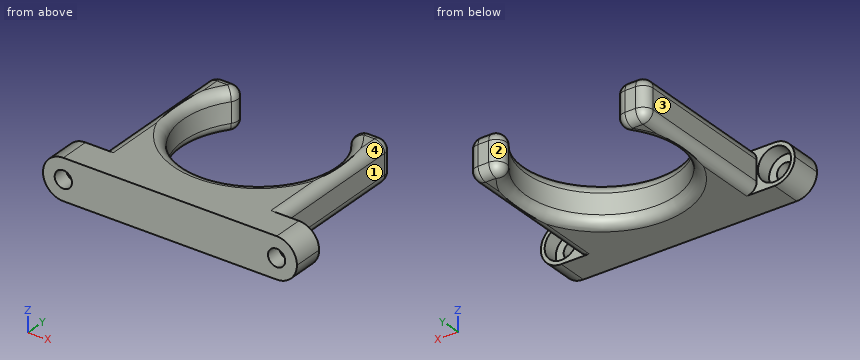
```python
from build123d import *

# Parameters (mm, degrees)
F1_DEPTH             = 8
F4_D                 = 3.4
F4_CBORE_D           = 6.5
F4_CBORE_DEPTH       = 3
F4_ON_F3_D           = 3.4
F4_ON_F3_CBORE_D     = 6.5
F4_ON_F3_CBORE_DEPTH = 3
F5_T1_DEPTH          = 2.0779215299
F5_T3_DEPTH          = 28
F5_T5_DEPTH          = 2.0779215299
F5_T8_ANGLE          = 253.4876833877
F5_T10_ANGLE         = 253.4876833877
F5_T12_ANGLE         = 126.7438416939
F5_T14_ANGLE         = 126.7438416939
F5_T16_ANGLE         = 90
F5_T18_ANGLE         = 90
F5_T20_ANGLE         = 126.7438416939
F5_T22_ANGLE         = 126.7438416939
F5_T24_ANGLE         = 90
F5_T26_ANGLE         = 90
F6_R                 = 3.99999


# Not quite as in the source:
# - a fillet or chamfer that OpenCascade refuses, or shapes differently, is made with other operations: its cross-section is extruded or revolved along the edge and cut away or added
# - a fillet or chamfer is up to 0.001 mm smaller than in the source, because OpenCascade refuses the exact size


with BuildPart() as f1:
    # F0 (on Top) → F1 (new body)
    with BuildSketch(Plane.XY):
        Polygon((-25, 6), (-25, 0), (25, 0), (25, 6), (17.5, 6), (-17.5, 6), align=None)
        with BuildLine():
            Line((-17.5, 34), (-17.5, 6))
            Line((-17.5, 6), (17.5, 6))
            Line((17.5, 6), (17.5, 34))
            ThreePointArc((17.5, 34), (16.9142135624, 35.4142135624), (15.5, 36))
            Line((15.5, 36), (13.4220784701, 36))
            ThreePointArc((13.4220784701, 36), (11.634209081, 34.896394471), (11.8194422349, 32.8035230476))
            ThreePointArc((11.8194422349, 32.8035230476), (0, 9.229505524), (-11.8194422349, 32.8035230476))
            ThreePointArc((-11.8194422349, 32.8035230476), (-11.634209081, 34.896394471), (-13.4220784701, 36))
            Line((-13.4220784701, 36), (-15.5, 36))
            ThreePointArc((-15.5, 36), (-16.9142135624, 35.4142135624), (-17.5, 34))
        make_face()
    extrude(amount=F1_DEPTH)

    # F4 (through all)
    with Locations(Plane(origin=(0, 6, 0), x_dir=(-1, 0, 0), z_dir=(0, 1, 0))):
        with Locations((-21, 4)):
            CounterBoreHole(F4_D / 2, F4_CBORE_D / 2, F4_CBORE_DEPTH)

    # F4 on F3 (through all)
    with Locations(Plane(origin=(0, 6, 0), x_dir=(-1, 0, 0), z_dir=(0, 1, 0))):
        with Locations((21, 4)):
            CounterBoreHole(F4_ON_F3_D / 2, F4_ON_F3_CBORE_D / 2, F4_ON_F3_CBORE_DEPTH)

    # F5: fillet of radius 2 on 2 edges, made by hand

    # F5_s2 → F5_t1 (cut)
    with BuildSketch(Plane.YZ.offset(-15.5)):
        with BuildLine():
            ThreePointArc((34, 8), (35.4142135624, 7.4142135624), (36, 6))
            Line((36, 6), (36, 8))
            Line((36, 8), (34, 8))
        make_face()
        with BuildLine():
            ThreePointArc((34, 0), (35.4142135624, 0.5857864376), (36, 2))
            Line((36, 2), (36, 0))
            Line((36, 0), (34, 0))
        make_face()
    extrude(amount=F5_T1_DEPTH, mode=Mode.SUBTRACT)

    # F5_s4 → F5_t3 (cut)
    with BuildSketch(Plane.XZ.offset(-34)):
        with BuildLine():
            ThreePointArc((-15.5, 8), (-16.9142135624, 7.4142135624), (-17.5, 6))
            Line((-17.5, 6), (-17.5, 8))
            Line((-17.5, 8), (-15.5, 8))
        make_face()
        with BuildLine():
            ThreePointArc((15.5, 8), (16.9142135624, 7.4142135624), (17.5, 6))
            Line((17.5, 6), (17.5, 8))
            Line((17.5, 8), (15.5, 8))
        make_face()
        with BuildLine():
            ThreePointArc((-15.5, 0), (-16.9142135624, 0.5857864376), (-17.5, 2))
            Line((-17.5, 2), (-17.5, 0))
            Line((-17.5, 0), (-15.5, 0))
        make_face()
        with BuildLine():
            ThreePointArc((15.5, 0), (16.9142135624, 0.5857864376), (17.5, 2))
            Line((17.5, 2), (17.5, 0))
            Line((17.5, 0), (15.5, 0))
        make_face()
    extrude(amount=F5_T3_DEPTH, mode=Mode.SUBTRACT)

    # F5_s6 → F5_t5 (cut)
    with BuildSketch(Plane.YZ.offset(13.4220784701)):
        with BuildLine():
            ThreePointArc((34, 8), (35.4142135624, 7.4142135624), (36, 6))
            Line((36, 6), (36, 8))
            Line((36, 8), (34, 8))
        make_face()
        with BuildLine():
            ThreePointArc((34, 0), (35.4142135624, 0.5857864376), (36, 2))
            Line((36, 2), (36, 0))
            Line((36, 0), (34, 0))
        make_face()
    extrude(amount=F5_T5_DEPTH, mode=Mode.SUBTRACT)

    # F5_s7 → F5_t8 (revolve, cut)
    with BuildSketch(Plane(origin=(-11.4952792826, 15.3974976921, 0), x_dir=(0, 0, 1), z_dir=(-0.5982384762, 0.8013181176, 0))):
        with BuildLine():
            ThreePointArc((0, 31.0954628442), (0.5857864376, 29.6812492818), (2, 29.0954628442))
            Line((2, 29.0954628442), (0, 29.0954628442))
            Line((0, 29.0954628442), (0, 31.0954628442))
        make_face()
    revolve(axis=Axis((0, 23.979505524, 0), (0, 0, -1)), revolution_arc=F5_T8_ANGLE, mode=Mode.SUBTRACT)

    # F5_s9 → F5_t10 (revolve, cut)
    with BuildSketch(Plane(origin=(-11.4952792826, 15.3974976921, 0), x_dir=(0, 0, 1), z_dir=(-0.5982384762, 0.8013181176, 0))):
        with BuildLine():
            ThreePointArc((8, 31.0954628442), (7.4142135624, 29.6812492818), (6, 29.0954628442))
            Line((6, 29.0954628442), (8, 29.0954628442))
            Line((8, 29.0954628442), (8, 31.0954628442))
        make_face()
    revolve(axis=Axis((0, 23.979505524, 8), (0, 0, -1)), revolution_arc=F5_T10_ANGLE, mode=Mode.SUBTRACT)

    # F5_s11 → F5_t12 (revolve, cut)
    with BuildSketch(Plane.YZ.offset(13.4220784701)):
        with BuildLine():
            ThreePointArc((34, 8), (35.4142135624, 7.4142135624), (36, 6))
            Line((36, 6), (36, 8))
            Line((36, 8), (34, 8))
        make_face()
    revolve(axis=Axis((13.4220784701, 34, 8), (0, 0, 1)), revolution_arc=F5_T12_ANGLE, mode=Mode.SUBTRACT)

    # F5_s13 → F5_t14 (revolve, cut)
    with BuildSketch(Plane(origin=(11.4952792826, 15.3974976921, 0), x_dir=(0, 0, 1), z_dir=(-0.5982384762, -0.8013181176, 0))):
        with BuildLine():
            ThreePointArc((8, 31.0954628442), (7.4142135624, 29.6812492818), (6, 29.0954628442))
            Line((6, 29.0954628442), (8, 29.0954628442))
            Line((8, 29.0954628442), (8, 31.0954628442))
        make_face()
    revolve(axis=Axis((-13.4220784701, 34, 8), (0, 0, 1)), revolution_arc=F5_T14_ANGLE, mode=Mode.SUBTRACT)

    # F5_s15 → F5_t16 (revolve, cut)
    with BuildSketch(Plane.YZ.offset(-15.5)):
        with BuildLine():
            ThreePointArc((34, 8), (35.4142135624, 7.4142135624), (36, 6))
            Line((36, 6), (36, 8))
            Line((36, 8), (34, 8))
        make_face()
    revolve(axis=Axis((-15.5, 34, 8), (0, 0, 1)), revolution_arc=F5_T16_ANGLE, mode=Mode.SUBTRACT)

    # F5_s17 → F5_t18 (revolve, cut)
    with BuildSketch(Plane.XZ.offset(-34)):
        with BuildLine():
            ThreePointArc((15.5, 8), (16.9142135624, 7.4142135624), (17.5, 6))
            Line((17.5, 6), (17.5, 8))
            Line((17.5, 8), (15.5, 8))
        make_face()
    revolve(axis=Axis((15.5, 34, 8), (0, 0, 1)), revolution_arc=F5_T18_ANGLE, mode=Mode.SUBTRACT)

    # F5_s19 → F5_t20 (revolve, cut)
    with BuildSketch(Plane.YZ.offset(13.4220784701)):
        with BuildLine():
            ThreePointArc((34, 0), (35.4142135624, 0.5857864376), (36, 2))
            Line((36, 2), (36, 0))
            Line((36, 0), (34, 0))
        make_face()
    revolve(axis=Axis((13.4220784701, 34, 0), (0, 0, 1)), revolution_arc=F5_T20_ANGLE, mode=Mode.SUBTRACT)

    # F5_s21 → F5_t22 (revolve, cut)
    with BuildSketch(Plane(origin=(11.4952792826, 15.3974976921, 0), x_dir=(0, 0, 1), z_dir=(-0.5982384762, -0.8013181176, 0))):
        with BuildLine():
            ThreePointArc((0, 31.0954628442), (0.5857864376, 29.6812492818), (2, 29.0954628442))
            Line((2, 29.0954628442), (0, 29.0954628442))
            Line((0, 29.0954628442), (0, 31.0954628442))
        make_face()
    revolve(axis=Axis((-13.4220784701, 34, 0), (0, 0, 1)), revolution_arc=F5_T22_ANGLE, mode=Mode.SUBTRACT)

    # F5_s23 → F5_t24 (revolve, cut)
    with BuildSketch(Plane.YZ.offset(-15.5)):
        with BuildLine():
            ThreePointArc((34, 0), (35.4142135624, 0.5857864376), (36, 2))
            Line((36, 2), (36, 0))
            Line((36, 0), (34, 0))
        make_face()
    revolve(axis=Axis((-15.5, 34, 0), (0, 0, 1)), revolution_arc=F5_T24_ANGLE, mode=Mode.SUBTRACT)

    # F5_s25 → F5_t26 (revolve, cut)
    with BuildSketch(Plane.XZ.offset(-34)):
        with BuildLine():
            ThreePointArc((15.5, 0), (16.9142135624, 0.5857864376), (17.5, 2))
            Line((17.5, 2), (17.5, 0))
            Line((17.5, 0), (15.5, 0))
        make_face()
    revolve(axis=Axis((15.5, 34, 0), (0, 0, 1)), revolution_arc=F5_T26_ANGLE, mode=Mode.SUBTRACT)

    # F6 (radius 4 in the source; OpenCascade refuses exactly that, so slightly less here)
    f6_edges = [f1.edges().sort_by_distance(p)[0] for p in [
        (-25, 3, 0),
        (-25, 3, 8),
        (25, 3, 0),
        (25, 3, 8),
    ]]
    fillet(f6_edges, radius=F6_R)


solid = f1.part
```
Part model, mm, in its own coordinate system. Face numbers are marked on the shaded views. A direction names the side the tool comes from. Round coordinates to 2 decimals unless told otherwise and drop trailing zeros. Loops run counter-clockwise (first coordinate to the right, second up) from the corner with the lowest first, then second, coordinate; pieces in that order, holes last.
1. Drill centre lines: line 1 along Z through (x, y) = (21, 5); line 2 along Y through (x, z) = (-19, 7.5); line 3 along X through (y, z) = (24, 5.75). Where is each one in solid material? Low to high.
Solutions:
line 1: z = 0 to 0.75, 7.25 to 8
line 2: y = 0 to 6
line 3: x = -17.5 to -14.75, 14.75 to 17.5
2. 3-axis set-ups, long thin cutter, end or side, ignore diameter. For the marked faces 1, 2, 3 and 4: which of +Z, -Z, +X, -X, +Y, -Y reach the whole face in a straight line?
Solutions:
face 1: +Z, -Z, +X, +Y
face 2: +Z, -Z
face 3: +Z, -Z, -X, +Y
face 4: +Z, +X, +Y
3. Slice it at B-B (x = 22). Give the cut face in (y, z), and give its area (3 significant figures).
Solutions:
outline: (0, 0.13) - (6, 0.13) - (6, 0.91) - (3, 0.91) - (3, 2.63) - (0, 2.63) - close; (0, 5.37) - (3, 5.37) - (3, 7.09) - (6, 7.09) - (6, 7.87) - (0, 7.87) - close
area: 19.7 mm2
4. Flat gauge pins, fed straight in: pin 1 (1 mm diameter, centred on y = 14, z = 1.5, fed in from -X); pin 2 (12 mm diameter, centred on x = 3, y = 13, fed in from +Z); pin 3 (4 mm diameter, centred on x = 21, z = 4, fed in from +Y); pin 4 (3 mm diameter, centred on y = 4, z = 1.5, fed in from -X). Where does each tip first touch, or does it go through?
Solutions:
pin 1: stops at x = -17.5
pin 2: stops at z = 8
pin 3: stops at y = 3
pin 4: stops at x = -24.87
5. Slice it at A-A (x = 0). Give the cut face in (y, z).
Solutions:
outline: (0, 0) - (7.23, 0) arc R2 ccw to (9.23, 2) - (9.23, 6) arc R2 ccw to (7.23, 8) - (0, 8) - close
